Verification items for this drawing (mm, ordinates from the low corner). A direction names the side the tool comes from. Round coordinates to 2 decimals unless told otherwise and drop trailing zeros. Loops run counter-clockwise (first coordinate to the right, second up) from the corner with the lowest first, then second, coordinate; pieces in that order, holes last. Notation, with made-up numbers: M 47,-7 L 106,-7 A23 ccw 106,3 Z; hole C 82,76.5 d11. An arc over 180 degrees is marked long. Use one line per item in the form item = value. Start each with the question number.
1. Set-up check for the marked faces 4, 5, 6, 7 and 8: record each of +Z, -Z, +X, -X, +Y, -Y from which the full face is reachable in a straight line by a thin tool's end or side.
2. Cross-section at D-D (z = 5.75). Record the boundary of the cut face in (x, y), then the cut area to 3 significant figures.
3. Cross-section at A-A (y = 1.25). Record the boundary of the cut face in (x, z), then the cut area to 3 significant figures.
4. Cross-section at B-B (y = 4.75). Record the boundary of the cut face in (x, z), then the cut area to 3 significant figures.
5. Cross-section at C-C (x = 2.5). Record the boundary of the cut face in (y, z).
6. Draft check along Z on the marked faces 1, 2 and 3. Enter one of: pulls with the +Z half, pulls with the -Z half, needs draft (parallel to the pull), parting line crosses it, or undercut.
7. Go/stop test with flat-tipped pins: pin 1 (6 mm diameter, centred on x = 27, z = 7.5, fed in from +Y); pin 2 (1 mm diameter, centred on y = 10.5, z = 9.5, fed in from +X); pin 3 (3 mm diameter, centred on x = 17, z = 3.5, fed in from -Y). Record where each tip stops, or that it passes through.
8. Material ranges on line 1 (X direction, y = 12.5, z = 3); line 2 (Z direction, x = 9.49, y = 12.7); line 3 (X direction, y = 10.25, z = 3), recorded low to high.
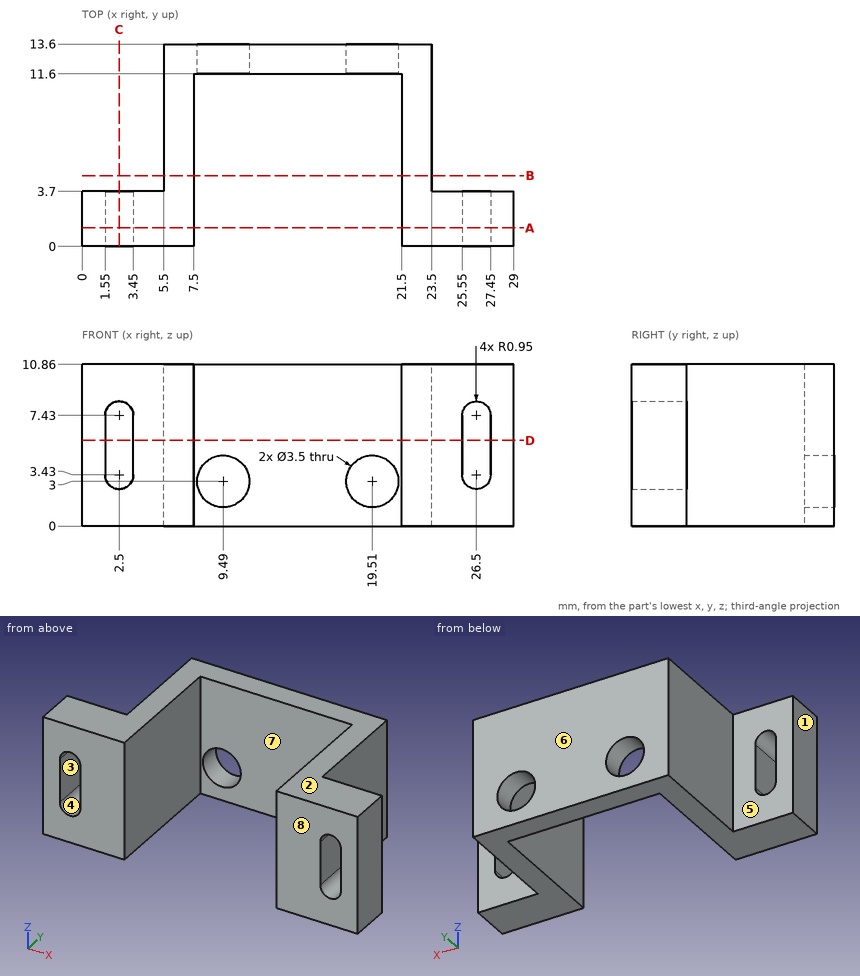
Reported:
q1.face_4 = +Y, -Y
q1.face_5 = +Z, -Z, -X, +Y
q1.face_6 = +Z, -Z, +X, -X, +Y
q1.face_7 = +Z, -Z, -Y
q1.face_8 = +Z, -Z, +X, -X, -Y
q2.outline = M 0,0 L 1.55,0 L 1.55,3.7 L 0,3.7 Z; M 3.45,0 L 7.5,0 L 7.5,11.6 L 21.5,11.6 L 21.5,0 L 25.55,0 L 25.55,3.7 L 23.5,3.7 L 23.5,13.6 L 5.5,13.6 L 5.5,3.7 L 3.45,3.7 Z; M 27.45,0 L 29,0 L 29,3.7 L 27.45,3.7 Z
q2.area = 109 mm²
q3.outline = M 0,0 L 7.5,0 L 7.5,10.86 L 0,10.86 Z; M 21.5,0 L 29,0 L 29,10.86 L 21.5,10.86 Z; hole M 1.55,3.43 A0.95 ccw 3.45,3.43 L 3.45,7.43 A0.95 ccw 1.55,7.43 Z; hole M 25.55,3.43 A0.95 ccw 27.45,3.43 L 27.45,7.43 A0.95 ccw 25.55,7.43 Z
q3.area = 142 mm²
q4.outline = M 5.5,0 L 7.5,0 L 7.5,10.86 L 5.5,10.86 Z; M 21.5,0 L 23.5,0 L 23.5,10.86 L 21.5,10.86 Z
q4.area = 43.4 mm²
q5.outline = M 0,0 L 3.7,0 L 3.7,2.48 L 0,2.48 Z; M 0,8.38 L 3.7,8.38 L 3.7,10.86 L 0,10.86 Z
q6.face_1 = needs draft
q6.face_2 = pulls with the +Z half
q6.face_3 = undercut
q7.pin_1 = 3.7
q7.pin_2 = 23.5
q7.pin_3 = 11.6
q8.line_1 = 5.5 to 7.74, 11.24 to 17.76, 21.26 to 23.5
q8.line_2 = 0 to 1.25, 4.75 to 10.86
q8.line_3 = 5.5 to 7.5, 21.5 to 23.5
